Build history of the part. All positions in model axes, mm. A direction names the side the tool comes from. Round coordinates to 2 decimals unless told otherwise and drop trailing zeros. Order: outer loops, then holes, each group sorted by start corner. A loop starts at its lowest first (then second) coordinate and runs counter-clockwise, first axis right, second up. Notation, with made-up numbers: M -21.75,-4.5 L 30.25,-4.5 A21 cw 30.25,25.5 Z; hole C 57.5,59.25 d9. An arc over 180 degrees is marked long. Use CSV: the item, a comma, the result in double quotes.
from build123d import *

# Parameters (mm, degrees)
F0_W     = 124.614488
F0_H     = 65.524992
F1_DEPTH = 124.46


with BuildPart() as f1:
    # F0 (on Front) → F1 (new body)
    with BuildSketch(Plane.XZ):
        with Locations((-40.518718, 1.739735)):
            Rectangle(F0_W, F0_H)
        Polygon((21.788526, -31.022761), (-102.825962, -31.022761), (-110.431544, -36.873206), (137.042314, -36.873206), (127.681583, -31.022761), (121.282354, -31.022761), (77.989712, -31.022761), align=None)
        Polygon((91.764651, 57.09333), (77.989712, -31.022761), (121.282354, -31.022761), (112.919003, 57.09333), align=None)
        with BuildLine():
            Line((127.681583, -31.022761), (137.042314, -36.873206))
            ThreePointArc((137.042314, -36.873206), (180.593446, 4.995028), (131.191865, 39.76763))
            ThreePointArc((131.191865, 39.76763), (123.821562, 38.078823), (127.681583, 31.577002))
            ThreePointArc((127.681583, 31.577002), (172.372699, 0.277121), (127.681583, -31.022761))
        make_face()
    extrude(amount=F1_DEPTH)


solid = f1.part
(1) Cut at B-B, the plane x = 145.5. Give the cut face in (y, z), and give its area (3 significant figures).
Answer block:
outline,"M -124.46,-36.94 L 0,-36.94 L 0,-32.4 L -124.46,-32.4 Z; M -124.46,32.96 L 0,32.96 L 0,40.97 L -124.46,40.97 Z"
area,"1,560 mm²"
(2) Drop flat-ended pins along their axis: pin 1 (3 mm diameter, centred on x = 125, y = -78, fed in from +Z); pin 2 (19.5 mm diameter, centred on y = -38, z = -9.5, fed in from +X); pin 3 (5 mm diameter, centred on y = -88, z = 32.5, fed in from +X). Give the stop position or say it passes through.
Answer block:
pin 1,"stops at z = 40.62"
pin 2,"stops at x = 180.67"
pin 3,"stops at x = 168.94"
(3) Two-plate mould, pull along X, no slides. Class faces 5 (the face through (-41, -61, 34.502)), 6 (the face through (84.974, -61.359, 13.652)), 7 (the face through (-106.58, -61.36, -33.91)), 8 (the face through (117.16, -61.36, 12.42)): released by +X, released by -X, zero draft, split by the parting line, or undercut.
Answer block:
face 5,"zero draft"
face 6,"undercut"
face 7,"released by -X"
face 8,"undercut"
(4) Cut at A-A, the plane z = 10. Give the cut face in (x, y), and give its area (3 significant figures).
Answer block:
outline,"M -102.83,-124.46 L 21.79,-124.46 L 21.79,0 L -102.83,0 Z; M 84.4,-124.46 L 117.39,-124.46 L 117.39,0 L 84.4,0 Z; M 170.92,-124.46 L 179.88,-124.46 L 179.88,0 L 170.92,0 Z"
area,"20,700 mm²"
(5) Cut at D-D, the plane z = -7. Give the cut face in (x, y).
Answer block:
outline,"M -102.83,-124.46 L 21.79,-124.46 L 21.79,0 L -102.83,0 Z; M 81.75,-124.46 L 119,-124.46 L 119,0 L 81.75,0 Z; M 171.57,-124.46 L 179.65,-124.46 L 179.65,0 L 171.57,0 Z"
(6) Wall check: line 1 (X direction, y = -19.5, z = 7); line 2 (X direction, y = -25, z = 29); line 3 (Z direction, x = -8.5, y = -91.5). Give the ranges that are in metal, low to high. Write a range as from..to.
Answer block:
line 1,"x = -102.83..21.79, 83.93..117.67, 171.69..180.39"
line 2,"x = -102.83..21.79, 87.37..115.59, 155.93..169.92"
line 3,"z = -36.87..34.5"
(7) Tool access for faces 1 (the face through (-102.826, -61, 1)), 2 (the face through (21.789, -61, 1)), 3 (the face through (125, -61, -31.023)), 4 (the face through (12, -61, -36.873)): list every direction of +Z, -Z, +X, -X, +Y, -Y with a clear straight run to the whole face (end or side of a thin tool).
Answer block:
face 1,"+Z, -X, +Y, -Y"
face 2,"+Z, +Y, -Y"
face 3,"+Y, -Y"
face 4,"-Z, -X, +Y, -Y"
(8) Cut at C-C, the plane x = -63. Give the cut face in (y, z), and give its area (3 significant figures).
Answer block:
outline,"M -124.46,-36.87 L 0,-36.87 L 0,34.5 L -124.46,34.5 Z"
area,"8,880 mm²"
